Here's the drawing with two shaded views (mm, measured from the low corner). I have some questions. A direction names the side the tool comes from. Round coordinates to 2 decimals unless told otherwise and drop trailing zeros. Write each loop counter-clockwise with the first axis right and the second up, starting at its lowest first coordinate (ties: lowest second). Pieces come first, ordered by that corner, then holes. Notation, with made-up numbers: (-6.75, -20.5) - (7.25, -20.5) arc R32 ccw to (7.25, 16.5) - close; hole circle Ø5 at (-7, -7.5). An arc over 180 degrees is marked (long way). Return JSON: item names as keys, results as strings. Group by question number.
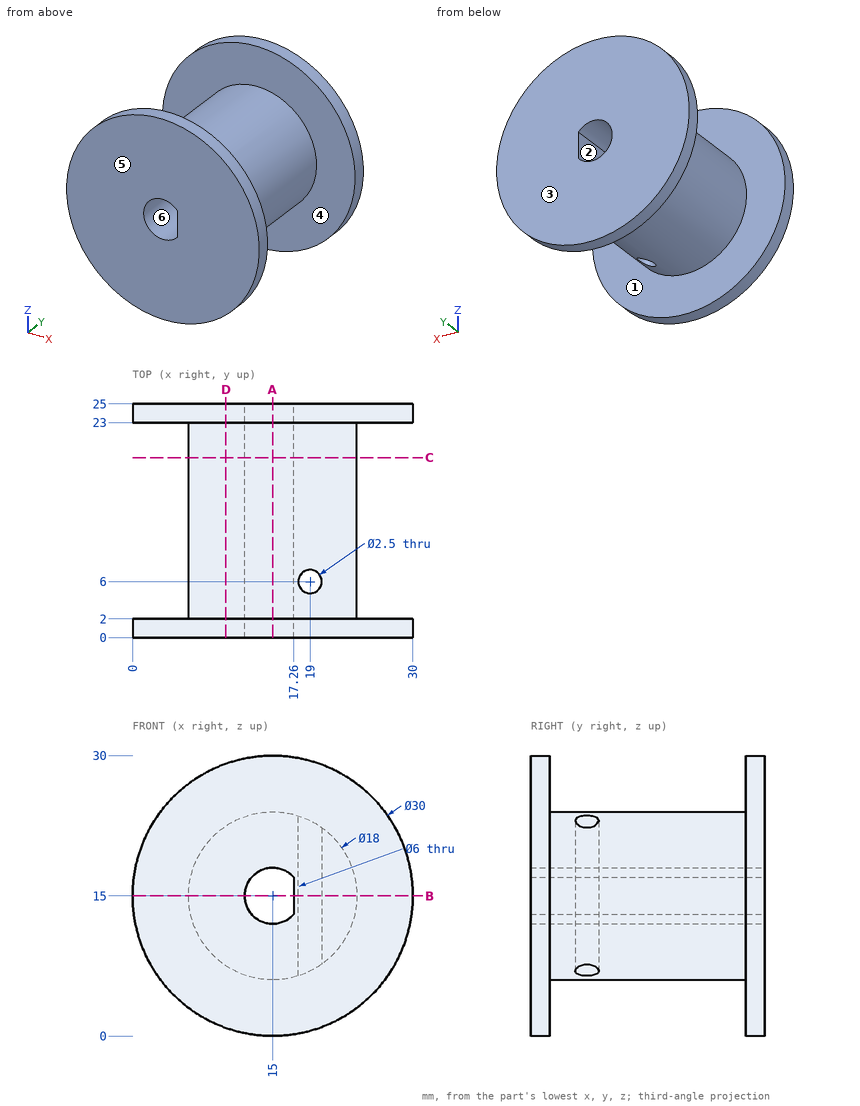
1) I need wall thicknesses on line 1 along Y through (x, z) = (26.5, 20); line 2 along Y through (x, z) = (19, 10.5); line 3 along X through (y, z) = (22.5, 14.75). Which ranges of each line are inside material? Lowest first, please.
2) Imagine slicing it at C-C (y = 19.25). Please give me the cut outline in (x, z), plus the area to 3 significant figures.
3) If we mould it in two halves opening along Y, with no side actions, what happens to the marked faces 4, 5 and 6? For each: released by +Y, released by -Y, zero draft, split by the parting line, or undercut.
4) Will these pins go through, and if not, where does the flat tip stop? pin 1 Ø2 at (x, y) = (23, 3.5) entering from -Z; pin 2 Ø8 at (x, y) = (24, 18) entering from -Z; pin 3 Ø3 at (x, y) = (19, 6) entering from +Z; pin 4 Ø10 at (x, y) = (17.5, 3.5) entering from +Z.
5) Imagine slicing it at B-B (z = 15). Please give me the cut outline in (x, y).
6) For the marked faces 1, 2 and 3, which set-ups out of +Z, -Z, +X, -X, +Y, -Y let a thin tool reach every point of the face, with its end or its side?
7) Imagine slicing it at D-D (x = 10). Please give me the cut outline in (y, z).
8) Imagine slicing it at A-A (x = 15). Please give me the cut outline in (y, z).
Results found:
{
 "1": {"line 1": "y = 0 to 2, 23 to 25", "line 2": "y = 0 to 4.75, 7.25 to 25", "line 3": "x = 6 to 12.01, 17.26 to 24"},
 "2": {"outline": "circle Ø18 at (15, 15); hole (17.26, 13.03) - (17.26, 16.97) arc R3 ccw (long way) to start", "area": "228 mm²"},
 "3": {"face 4": "undercut", "face 5": "released by -Y", "face 6": "zero draft"},
 "4": {"pin 1": "stops at z = 9.34", "pin 2": "stops at z = 7.52", "pin 3": "stops at z = 23.65", "pin 4": "stops at z = 30"},
 "5": {"outline": "(0, 0) - (12, 0) - (12, 25) - (0, 25) - (0, 23) - (6, 23) - (6, 2) - (0, 2) - close; (17.26, 0) - (30, 0) - (30, 2) - (24, 2) - (24, 23) - (30, 23) - (30, 25) - (17.26, 25) - close; hole circle Ø2.5 at (19, 6)"},
 "6": {"face 1": "none", "face 2": "+Y, -Y", "face 3": "+Z, -Z, +X, -X, +Y"},
 "7": {"outline": "(0, 0.86) - (2, 0.86) - (2, 7.52) - (23, 7.52) - (23, 0.86) - (25, 0.86) - (25, 29.14) - (23, 29.14) - (23, 22.48) - (2, 22.48) - (2, 29.14) - (0, 29.14) - close"},
 "8": {"outline": "(0, 0) - (2, 0) - (2, 6) - (23, 6) - (23, 0) - (25, 0) - (25, 12) - (0, 12) - close; (0, 18) - (25, 18) - (25, 30) - (23, 30) - (23, 24) - (2, 24) - (2, 30) - (0, 30) - close"}
}
